Autodesk Inventor part; units mm, degrees
ref_plane "YZ Plane" through (0, 0, 0) normal (1, 0, 0) x (0, 1, 0)
ref_plane "XZ Plane" through (0, 0, 0) normal (0, 1, 0) x (-1, 0, 0)
ref_plane "XY Plane" through (0, 0, 0) normal (0, 0, 1) x (1, 0, 0)
sketch "Sketch1" plane through (0, 0, 0) normal (0, 0, 1) x (1, 0, 0)
  line L0 (186.7379, 130.6481) -> (186.7379, -66.2019)
  line L1 (186.7379, -66.2019) -> (-194.2621, -66.2019)
  line L2 (-194.2621, -66.2019) -> (-194.2621, 130.6481)
  line L3 (-194.2621, 130.6481) -> (-130.7621, 130.6481)
  line L4 (186.7379, 130.6481) -> (123.2379, 130.6481)
  arc A0 (-130.7621, 130.6481) -> (123.2379, 130.6481) centre (-3.7621, 214.8904) ccw
  point P0 (0, 0)
  dimension "d0" = 381
  dimension "d1" = 196.85
  dimension "d41" = 63.5
  dimension "d42" = 63.5
  dimension "d43" = 152.4
extrude "Extrusion1" add sketch "Sketch1" along normal blind 6.35
hole "Hole2" at (-137.1121, 54.4481, 6.35) direction (0, 0, -1) diameter 63.5 end through all
hole "Hole3" at (129.5879, 54.4481, 6.35) direction (0, 0, -1) diameter 63.5 end through all
hole "Hole4" at (-181.5621, -53.5019, 6.35) direction (0, 0, -1) diameter 3.175 end through all
hole "Hole5" at (174.0379, -53.5019, 6.35) direction (0, 0, -1) diameter 3.175 end through all
pattern_linear "Rectangular Pattern4" count 6 spacing 25.4 along (0, 1, 0) of "Hole4"
pattern_linear "Rectangular Pattern5" count 6 spacing 25.4 along (0, 1, 0) of "Hole5"
pattern_linear "Rectangular Pattern6" count 4 spacing 25.4 along (-1, 0, 0) count 2 spacing 25.4 along (0, 1, 0) of "Hole5"
hole "Hole6" at (-181.5621, 103.6479, 6.35) direction (0, 0, -1) diameter 3.175 end through all
pattern_linear "Rectangular Pattern7" count 20 spacing 25.4 along (1, 0, 0) of "Hole6"
hole "Hole7" at (-133.7621, -48.2019, 6.35) direction (0, 0, -1) diameter 6.35 end through all
pattern_linear "Rectangular Pattern8" count 2 spacing 36 along (0, 1, 0) of "Hole7"
hole "Hole8" at (-32.2621, -48.2019, 6.35) direction (0, 0, -1) diameter 6.35 end through all
pattern_linear "Rectangular Pattern9" count 2 spacing 36 along (0, 1, 0) of "Hole8"
hole "Hole9" at (64.2379, -48.2019, 6.35) direction (0, 0, -1) diameter 6.35 end through all
pattern_linear "Rectangular Pattern10" count 2 spacing 36 along (0, 1, 0) of "Hole9"
properties part number "Devant - Bas Rammasse-Balle"
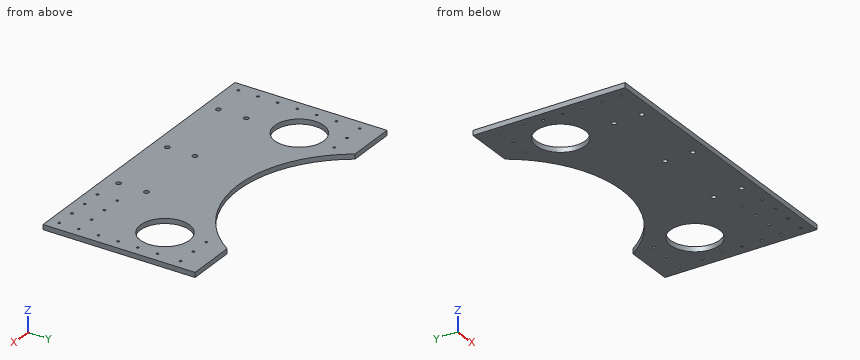
Geometry check sheet. Reference: the model listing, model coordinates, mm. Coordinates: 2 decimals unless noted, no trailing zeros. Write each loop counter-clockwise with the first axis right and the second up, starting at its lowest first coordinate (ties: lowest second). Pieces come first, ordered by that corner, then holes. Notation, with made-up numbers: M -11,23.5 L 27,23.5 A18 cw 27,49.5 Z; hole C -9,0 d3. An arc over 180 degrees is marked long. One line per item, written item: value. Start each with the question number.
(1) Sectioned sample at C-C, the plane z = 3.25. State how many separate pieces and enclosed holes the cut face has, and give its area (3 significant figures).
(2) Scan lines: line 1 along X through (y, z) = (52.5, 4); line 2 along X through (y, z) = (-1.5, 5.5) (3 decimals); line 3 along X through (y, z) = (99, 4.75). Record each from-to range of solid material in increasing order. Write a range as [from, to].
(3) Sectioned sample at B-B, the plane x = -96.5. Enter the section's corners in (y, z).
(4) Sectioned sample at D-D, the plane x = 20.5. Enter the section's corners in (y, z), and give its area (3 significant figures).
(5) Sectioned sample at A-A, the plane y = 54.5. Enter the section's corners in (x, z), and give its area (3 significant figures).
Filled sheet:
1. separate pieces: 1
1. enclosed holes: 32
1. area: 56,100 mm²
2. line 1: [-194.26, -168.8], [-105.42, 97.9], [161.28, 186.74]
2. line 2: [-194.262, -182.599], [-180.525, 173.001], [175.075, 186.738]
2. line 3: [-194.26, -102.73], [95.21, 186.74]
3. outline: M -66.2,0 L 93.95,0 L 93.95,6.35 L -66.2,6.35 Z
4. outline: M -66.2,0 L 64.43,0 L 64.43,6.35 L -66.2,6.35 Z
4. area: 830 mm²
5. outline: M -194.26,0 L -168.86,0 L -168.86,6.35 L -194.26,6.35 Z; M -105.36,0 L 97.84,0 L 97.84,6.35 L -105.36,6.35 Z; M 161.34,0 L 186.74,0 L 186.74,6.35 L 161.34,6.35 Z
5. area: 1,610 mm²
